from build123d import *

# Parameters (mm, degrees)
F0_W      = 20.930506
F0_H      = 12.882103
F1_DEPTH  = 38.67383
F1_FACE_W = 20.930506
F1_FACE_H = 38.67383
F2_DEPTH  = 53.03582
F3_R      = 4.727267
F4_DEPTH  = 25.20039


with BuildPart() as f1:
    # F0 (on Front) → F1 (new body)
    with BuildSketch(Plane.XZ):
        with Locations((-29.003717, 19.335555)):
            Rectangle(F0_W, F0_H)
    extrude(amount=F1_DEPTH)

    # F1_face (on face) → F2 (join)
    with BuildSketch(Plane(origin=(-29.003717, -19.336915, 25.776606), x_dir=(1, 0, 0), z_dir=(0, 0, 1))):
        Rectangle(F1_FACE_W, F1_FACE_H)
    extrude(amount=F2_DEPTH)

    # F3 (on face) → F4 (cut)
    with BuildSketch(Plane.XZ.offset(38.67383)):
        with Locations((-25.014196, 44.345655)):
            Circle(F3_R)
    extrude(amount=-F4_DEPTH, mode=Mode.SUBTRACT)


solid = f1.part
The listing builds one solid part. Answer for the finished solid, in the listing's coordinates (mm). Give positions to 0.01 mm unless a question says otherwise; leave off trailing zeros. Write each loop counter-clockwise with the first axis right and the second up, starting at its lowest first coordinate (ties: lowest second). Pieces come first, ordered by that corner, then holes. Notation, with made-up numbers: (89.5, 50.5) - (147.5, 50.5) arc R6 cw to (147.5, 57.5) - close; hole circle Ø8 at (9.25, 15.5). An arc over 180 degrees is marked (long way). One line per question, with ' | ' between items. Start each with the question number.
1. Given P1, Ø3, axis at x = -22.5, z = 45, coming from the -Y side, flat-ended and moving along its own axis, determine where the tip first touches the part or whether it passes through.
2. Determine the mould class of faces 1 (the face through (-29, -19, 78.812)), 2 (the face through (-28.5, -26.25, 47.54)), 3 (the face through (-25, -13.473, 44)), 4 (the face through (-39.469, -19, 45)) for opening direction X: +X half, -X half, draft (parallel to the pull), parting line (faces both ways), or undercut.
3. Straight lines are drawn through the part: line 1 (Z direction, x = -25.25, y = -19.5); line 2 (Z direction, x = -28.75, y = -16); line 3 (X direction, y = -17.5, z = 40). For each, find the intervals that lie inside material, in ascending order.
4. Section A-A, the plane x = -27.5 is taken. Determine the outline of the cut face in (y, z).
5. Section B-B, the plane y = -29.5 is taken. Determine the outline of the cut face in (x, z), then the cut area to 3 significant figures.
6. Section C-C, the plane x = -21 is taken. Determine the outline of the cut face in (y, z).
Result:
1) P1: stops at y = -13.47
2) face 1: draft | face 2: undercut | face 3: undercut | face 4: -X half
3) line 1: z = 12.89 to 39.62, 49.07 to 78.81 | line 2: z = 12.89 to 41.45, 47.24 to 78.81 | line 3: x = -39.47 to -26.87, -23.15 to -18.54
4) outline: (-38.67, 12.89) - (0, 12.89) - (0, 78.81) - (-38.67, 78.81) - (-38.67, 48.37) - (-13.47, 48.37) - (-13.47, 40.32) - (-38.67, 40.32) - close
5) outline: (-39.47, 12.89) - (-18.54, 12.89) - (-18.54, 78.81) - (-39.47, 78.81) - close; hole circle Ø9.45 at (-25.01, 44.35) | area: 1,310 mm2
6) outline: (-38.67, 12.89) - (0, 12.89) - (0, 78.81) - (-38.67, 78.81) - (-38.67, 46.84) - (-13.47, 46.84) - (-13.47, 41.85) - (-38.67, 41.85) - close
